Autodesk Inventor part; units mm, degrees
ref_plane "YZ Plane" through (0, 0, 0) normal (1, 0, 0) x (0, 1, 0)
ref_plane "XZ Plane" through (0, 0, 0) normal (0, 1, 0) x (-1, 0, 0)
ref_plane "XY Plane" through (0, 0, 0) normal (0, 0, 1) x (1, 0, 0)
sketch "Sketch1" plane through (0, 0, 0) normal (0, 1, 0) x (-1, 0, 0)
  line L0 (101.0364, -60.995) -> (-18.9636, -60.995)
  line L1 (-18.9636, -60.995) -> (-18.9636, 59.005)
  line L2 (-18.9636, 59.005) -> (101.0364, 59.005)
  line L3 (101.0364, 59.005) -> (101.0364, -60.995)
  line L4 (93.1598, 54.938) -> (-8.3402, 54.938) construction
  line L5 (-8.3402, 54.938) -> (-8.3402, 1.138) construction
  line L6 (-8.3402, 1.138) -> (93.1598, 1.138) construction
  line L7 (93.1598, 1.138) -> (93.1598, 54.938) construction
  line L8 (92.9387, -1.5201) -> (30.3387, -1.5201) construction
  line L9 (30.3387, -1.5201) -> (30.3387, -58.6201) construction
  line L10 (30.3387, -58.6201) -> (92.9387, -58.6201) construction
  line L11 (92.9387, -58.6201) -> (92.9387, -1.5201) construction
  line L12 (27.7395, -7.49) -> (-15.5605, -7.49) construction
  line L13 (-15.5605, -7.49) -> (-15.5605, -50.79) construction
  line L14 (-15.5605, -50.79) -> (27.7395, -50.79) construction
  line L15 (27.7395, -50.79) -> (27.7395, -7.49) construction
  line L16 (65.0387, -49.7201) -> (62.2387, -49.7201) construction
  line L17 (62.2387, -49.7201) -> (62.2387, -52.5201) construction
  line L18 (62.2387, -52.5201) -> (65.0387, -52.5201) construction
  line L19 (65.0387, -52.5201) -> (65.0387, -49.7201) construction
  circle A0 centre (65.0387, -7.1201) radius 1.4
  circle A1 centre (63.6387, -51.1201) radius 1.4
  line L20 (92.1598, 53.938) -> (89.3598, 53.938) construction
  line L21 (89.3598, 53.938) -> (89.3598, 51.138) construction
  line L22 (89.3598, 51.138) -> (92.1598, 51.138) construction
  line L23 (92.1598, 51.138) -> (92.1598, 53.938) construction
  line L24 (-4.5402, 4.938) -> (-7.3402, 4.938) construction
  line L25 (-7.3402, 4.938) -> (-7.3402, 2.138) construction
  line L26 (-7.3402, 2.138) -> (-4.5402, 2.138) construction
  line L27 (-4.5402, 2.138) -> (-4.5402, 4.938) construction
  circle A2 centre (-5.9402, 3.538) radius 1.4
  circle A3 centre (90.7598, 52.538) radius 1.4
  line L28 (26.3395, -8.59) -> (23.5395, -8.59) construction
  line L29 (23.5395, -8.59) -> (23.5395, -11.39) construction
  line L30 (23.5395, -11.39) -> (26.3395, -11.39) construction
  line L31 (26.3395, -11.39) -> (26.3395, -8.59) construction
  line L32 (-11.3605, -46.89) -> (-14.1605, -46.89) construction
  line L33 (-14.1605, -46.89) -> (-14.1605, -49.69) construction
  line L34 (-14.1605, -49.69) -> (-11.3605, -49.69) construction
  line L35 (-11.3605, -49.69) -> (-11.3605, -46.89) construction
  line L36 (-11.3605, -8.59) -> (-14.1605, -8.59) construction
  line L37 (-14.1605, -8.59) -> (-14.1605, -11.39) construction
  line L38 (-14.1605, -11.39) -> (-11.3605, -11.39) construction
  line L39 (-11.3605, -11.39) -> (-11.3605, -8.59) construction
  line L40 (26.3395, -46.89) -> (23.5395, -46.89) construction
  line L41 (23.5395, -46.89) -> (23.5395, -49.69) construction
  line L42 (23.5395, -49.69) -> (26.3395, -49.69) construction
  line L43 (26.3395, -49.69) -> (26.3395, -46.89) construction
  circle A4 centre (24.9395, -9.99) radius 1.4
  circle A5 centre (24.9395, -48.29) radius 1.4
  circle A6 centre (-12.7605, -48.29) radius 1.4
  circle A7 centre (-12.7605, -9.99) radius 1.4
  circle A8 centre (24.9395, -9.99) radius 2.4
  circle A9 centre (24.9395, -48.29) radius 2.4
  circle A10 centre (-12.7605, -48.29) radius 2.4
  circle A11 centre (-12.7605, -9.99) radius 2.4
  circle A12 centre (63.6387, -51.1201) radius 2.4
  circle A13 centre (65.0387, -7.1201) radius 2.4
  circle A14 centre (-5.9402, 3.538) radius 2.4
  circle A15 centre (90.7598, 52.538) radius 2.4
  line L44 (-20.9636, 61.005) -> (103.0364, 61.005)
  line L45 (103.0364, 61.005) -> (103.0364, -62.995)
  line L46 (103.0364, -62.995) -> (-20.9636, -62.995)
  line L47 (-20.9636, -62.995) -> (-20.9636, 61.005)
  circle A16 centre (97.4742, -19.995) radius 1.4
  circle A17 centre (97.4742, 57.3306) radius 1.4
  circle A18 centre (53.0364, 57.3306) radius 1.4
  circle A19 centre (29.2299, -19.995) radius 1.4
  circle A20 centre (29.0364, 57.3306) radius 1.4
  dimension "d0" = 120
  dimension "d1" = 120
  dimension "d8" = 101.5
  dimension "d9" = 53.8
  dimension "d10" = 62.6
  dimension "d11" = 57.1
  dimension "d12" = 43.3
  dimension "d13" = 43.3
  dimension "d24" = 4.067
  dimension "d25" = 10.6234
  dimension "d27" = 10.205
  dimension "d28" = 3.403
  dimension "d29" = 2.3749
  dimension "d30" = 8.0977
  dimension "d39" = 2.8
  dimension "d40" = 2.8
  dimension "d41" = 6.1
  dimension "d42" = 2.8
  dimension "d43" = 2.8
  dimension "d44" = 2.8
  dimension "d45" = 2.8
  dimension "d46" = 1
  dimension "d47" = 1
  dimension "d48" = 1
  dimension "d49" = 1
  dimension "d50" = 2.8
  dimension "d51" = 2.8
  dimension "d52" = 2.8
  dimension "d53" = 2.8
  dimension "d54" = 2.8
  dimension "d55" = 2.8
  dimension "d56" = 2.8
  dimension "d57" = 2.8
  dimension "d58" = 1.4
  dimension "d59" = 1.1
  dimension "d60" = 1.4
  dimension "d61" = 1.1
  dimension "d62" = 1.1
  dimension "d63" = 1.4
  dimension "d64" = 1.1
  dimension "d65" = 1.4
  dimension "d66" = 4.8
  dimension "d67" = 4.8
  dimension "d68" = 4.8
  dimension "d69" = 4.8
  dimension "d70" = 4.8
  dimension "d71" = 4.8
  dimension "d72" = 4.8
  dimension "d73" = 4.8
  dimension "d74" = 124
  dimension "d75" = 124
  dimension "d76" = 2
  dimension "d77" = 2
  dimension "d144" = 44
  dimension "d145" = 2.8
  dimension "d146" = 41
  dimension "d148" = 2.8
  dimension "d149" = 2.8
  dimension "d150" = 50
  dimension "d154" = 2.8
  dimension "d155" = 50
extrude "Extrusion1" add sketch "Sketch1" against normal blind 2.5 contours L0 L1 L2 L3 | A0 | A1 | A2 | A3 | A4 | A5 | A6 | A7 | A8 | A9 | A10 | A11 | A12 | A13 | A14 | A15 | L44 L45 L46 L47 | A16 | A17 | A18 | A19 | A20
extrude "Extrusion2" add sketch "Sketch1" along normal blind 30 contours L44 L45 L46 L47
extrude "Extrusion3" add sketch "Sketch1" along normal blind 3 contours A15
extrude "Extrusion4" add sketch "Sketch1" along normal blind 3 contours A13
extrude "Extrusion5" add sketch "Sketch1" along normal blind 3 contours A12
extrude "Extrusion6" add sketch "Sketch1" along normal blind 3 contours A9
extrude "Extrusion7" add sketch "Sketch1" along normal blind 3 contours A8
extrude "Extrusion8" add sketch "Sketch1" along normal blind 3 contours A14
extrude "Extrusion9" add sketch "Sketch1" along normal blind 3 contours A11
extrude "Extrusion10" add sketch "Sketch1" along normal blind 3 contours A10
sketch "Sketch3" plane through (-103.0364, -2.5, -62.995) normal (-1, 0, 0) x (0, 0, 1)
  line L0 (122, 32.5) -> (2, 32.5)
  line L1 (2, 2.5) -> (122, 2.5)
  line L2 (10, 32.5) -> (114, 32.5)
  line L3 (114, 32.5) -> (114, 2.5)
  line L4 (114, 2.5) -> (10, 2.5)
  line L5 (10, 2.5) -> (10, 32.5)
  line L6 (0, 0) -> (0, 32.5)
  point P0 (62.995, 2.5)
  dimension "d98" = 104
  dimension "d99" = 10
extrude "Extrusion11" cut sketch "Sketch3" against normal blind 3
sketch "Sketch4" plane through (20.9636, -2.5, 61.005) normal (1, 0, 0) x (0, 0, -1)
  line L0 (122, 32.5) -> (2, 32.5)
  line L1 (10, 32.5) -> (114, 32.5)
  line L2 (114, 32.5) -> (114, 2.5)
  line L3 (114, 2.5) -> (10, 2.5)
  line L4 (10, 2.5) -> (10, 32.5)
  line L5 (0, 0) -> (0, 32.5)
  point P0 (61.005, 2.5)
  dimension "d102" = 104
  dimension "d103" = 10
extrude "Extrusion12" cut sketch "Sketch4" against normal blind 3
sketch "Sketch5" plane through (20.9636, -2.5, 61.005) normal (1, 0, 0) x (0, 0, -1)
  line L0 (3.7, 25.8817) -> (6.5, 25.8817) construction
  line L1 (6.5, 25.8817) -> (6.5, 23.0817) construction
  line L2 (6.5, 23.0817) -> (3.7, 23.0817) construction
  line L3 (3.7, 23.0817) -> (3.7, 25.8817) construction
  line L4 (3.7, 17.6669) -> (6.5, 17.6669) construction
  line L5 (6.5, 17.6669) -> (6.5, 14.8669) construction
  line L6 (6.5, 14.8669) -> (3.7, 14.8669) construction
  line L7 (3.7, 14.8669) -> (3.7, 17.6669) construction
  line L8 (10, 2.5) -> (10, 32.5)
  circle A0 centre (5.1, 24.8) radius 1.4
  circle A1 centre (5.1, 16.3) radius 1.4
  line L9 (117.5, 24.7669) -> (120.3, 24.7669) construction
  line L10 (0, 32.5) -> (10, 32.5)
  line L11 (117.5, 16.3) -> (120.3, 16.3) construction
  line L12 (114, 32.5) -> (114, 2.5)
  circle A2 centre (118.9, 24.8) radius 1.4
  circle A3 centre (118.9, 16.3) radius 1.4
  line L13 (114, 32.5) -> (124, 32.5)
  point P0 (61.005, 2.5)
  dimension "d106" = 2.8
  dimension "d107" = 2.8
  dimension "d108" = 2.8
  dimension "d109" = 2.8
  dimension "d110" = 3.5
  dimension "d111" = 3.5
  dimension "d112" = 8.5
  dimension "d115" = 7.7
  dimension "d120" = 7.7
  dimension "d121" = 8.5
  dimension "d122" = 2.8
  dimension "d123" = 2.8
  dimension "d124" = 4.9
  dimension "d125" = 4.9
  dimension "d126" = 4.9
  dimension "d127" = 4.9
extrude "Extrusion13" cut sketch "Sketch5" against normal blind 130
sketch "Sketch6" plane through (-103.0364, -2.5, 61.005) normal (0, 0, 1) x (1, 0, 0)
  line L0 (57, 19.5) -> (67, 19.5) construction
  line L1 (67, 19.5) -> (67, 9.5) construction
  line L2 (67, 9.5) -> (57, 9.5) construction
  line L3 (57, 9.5) -> (57, 19.5) construction
  line L4 (0, 32.5) -> (124, 32.5)
  line L5 (54.55, 28) -> (57.35, 28) construction
  line L6 (57.35, 28) -> (57.35, 25.2) construction
  line L7 (57.35, 25.2) -> (54.55, 25.2) construction
  line L8 (54.55, 25.2) -> (54.55, 28) construction
  line L9 (66.65, 25.1915) -> (69.45, 25.1915) construction
  line L10 (69.45, 25.1915) -> (69.45, 27.9915) construction
  line L11 (69.45, 27.9915) -> (66.65, 27.9915) construction
  line L12 (66.65, 27.9915) -> (66.65, 25.1915) construction
  line L13 (124, 0) -> (124, 32.5)
  line L14 (0, 0) -> (0, 32.5)
  circle A0 centre (55.95, 26.5915) radius 1.4
  circle A1 centre (68.05, 26.5915) radius 1.4
  circle A2 centre (62, 14.5) radius 5
  point P0 (103.0364, 2.5)
  dimension "d130" = 10
  dimension "d131" = 10
  dimension "d132" = 13
  dimension "d133" = 2.8
  dimension "d134" = 2.8
  dimension "d135" = 2.8
  dimension "d136" = 2.8
  dimension "d137" = 9.3
  dimension "d138" = 5.7
  dimension "d139" = 54.55
  dimension "d140" = 54.55
  dimension "d141" = 57
extrude "Extrusion14" cut sketch "Sketch6" against normal blind 130
extrude "Extrusion15" add sketch "Sketch1" along normal blind 26 contours A16 | A17 | A18 | A19
sketch "Sketch7" plane through (20.9636, -2.5, 61.005) normal (1, 0, 0) x (0, 0, -1)
  line L0 (2, 2.5) -> (2, 32.5)
  line L1 (10, 32.5) -> (10, 2.5)
  line L2 (2, 32.5) -> (10, 32.5)
  line L3 (10, 32.5) -> (10, 8.5)
  line L4 (10, 8.5) -> (2, 8.5)
  line L5 (2, 8.5) -> (2, 32.5)
  line L6 (122, 32.5) -> (114, 32.5)
  line L7 (122, 2.5) -> (122, 32.5)
  line L8 (114, 32.5) -> (122, 32.5)
  line L9 (122, 32.5) -> (122, 8.5)
  line L10 (122, 8.5) -> (114, 8.5)
  line L11 (114, 8.5) -> (114, 32.5)
  point P0 (61.005, 2.5)
  dimension "d156" = 24
  dimension "d157" = 24
extrude "Extrusion16" cut sketch "Sketch7" against normal blind 1
sketch "Sketch8" plane through (-103.0364, -2.5, -62.995) normal (-1, 0, 0) x (0, 0, 1)
  line L0 (2, 2.5) -> (2, 32.5)
  line L1 (10, 2.5) -> (10, 32.5)
  line L2 (2, 32.5) -> (10, 32.5)
  line L3 (10, 32.5) -> (10, 8.5)
  line L4 (10, 8.5) -> (2, 8.5)
  line L5 (2, 8.5) -> (2, 32.5)
  line L6 (114, 32.5) -> (124, 32.5)
  line L7 (122, 2.5) -> (122, 32.5)
  line L8 (114, 32.5) -> (122, 32.5)
  line L9 (122, 32.5) -> (122, 8.5)
  line L10 (122, 8.5) -> (114, 8.5)
  line L11 (114, 8.5) -> (114, 32.5)
  point P0 (62.995, 2.5)
  dimension "d160" = 24
  dimension "d161" = 24
extrude "Extrusion17" cut sketch "Sketch8" against normal blind 1
extrude "Extrusion18" cut sketch "Sketch1" against normal blind 1.5 contours A0 | A1 | A2 | A3 | A4 | A5 | A6 | A7
properties part number "Lower_Housing" material "Iron, Cast"
Design review of the part built by this model. Coordinates are the model's own, in mm. A direction names the side the tool comes from. Round coordinates to 2 decimals unless told otherwise and drop trailing zeros. Write each loop counter-clockwise with the first axis right and the second up, starting at its lowest first coordinate (ties: lowest second). Pieces come first, ordered by that corner, then holes. Notation, with made-up numbers: (2, -5.5) -> (12, -5.5) arc R19 cw to (12, 23.5) -> close; hole circle Ø5 at (55, 19). An arc over 180 degrees is marked (long way). Write item = value, one per line. Start each with the question number.
1) Take a section at A-A, the plane x = -84. State the section outline as (y, z) points (3 decimals), plus the area to 3 significant figures.
2) Clearance check with flat-ended pins moving along their axes: pin 1 (4 mm diameter, centred on y = 13, z = -58, fed in from +X); pin 2 (8 mm diameter, centred on x = -74.5, z = 39.5, fed in from +Y); pin 3 (5.5 mm diameter, centred on x = 13, z = -10.5, fed in from +Y); pin 4 (1.7 mm diameter, centred on x = -47.09, y = 24.09, fed in from +Z). State where each tip first meets the part, or that it passes through.
3) Wall thickness on probe 1 along Z at (x, y) = (-60, 4) (3 decimals); probe 2 along Z at (x, y) = (-92, 1) (3 decimals); probe 3 along X at (y, z) = (17.5, 54.5): over which ranges is each line inside the solid? List them lowest first. Write a range as from..to.
4) Take a section at B-B, the plane z = -3. State the section outline as (x, y) points, plus the area to 3 significant figures.
5) Mouldability with a two-part tool opening along Y and no side actions: class faces 1 (the face through (5.97, 3, 1.97)), 2 (the face through (19.471, 21.764, -59.188)), 3 (the face through (18.964, 15, 54)) as +Y half, -Y half, draft (parallel to the pull), parting line (faces both ways), or undercut.
6) Tool access review of faces 4 (the face through (12.94, 0.72, -49.68)), 5 (the face through (20.964, -1, -1)), 6 (the face through (-41, 30, -62)), 7 (the face through (19.964, 18, 55)), 8 (the face through (-27, 3, -10)): name each direction out of +Z, -Z, +X, -X, +Y, -Y from which nothing blocks a thin tool from reaching the whole face with its end or side.
Results list:
q1.outline = (-2.5, -62.995) -> (30, -62.995) -> (30, -60.995) -> (0, -60.995) -> (0, 59.005) -> (30, 59.005) -> (30, 61.005) -> (-2.5, 61.005) -> close
q1.area = 430 mm²
q2.pin_1 = 19.96
q2.pin_2 = 0
q2.pin_3 = 3
q2.pin_4 = through
q3.probe_1 = -62.995..-60.995, 59.005..61.005
q3.probe_2 = -62.995..-60.995, 50.483..51.888, 53.188..54.593, 59.005..61.005
q3.probe_3 = -102.04..-101.04, 18.96..19.96
q4.outline = (-103.04, -2.5) -> (20.96, -2.5) -> (20.96, 0) -> (-103.04, 0) -> close
q4.area = 310 mm²
q5.face_1 = +Y half
q5.face_2 = undercut
q5.face_3 = draft
q6.face_4 = +Y
q6.face_5 = +Z, -Z, +X, +Y, -Y
q6.face_6 = +Z, -Z, +X, -X, +Y
q6.face_7 = +X, +Y
q6.face_8 = +X, -X, +Y
